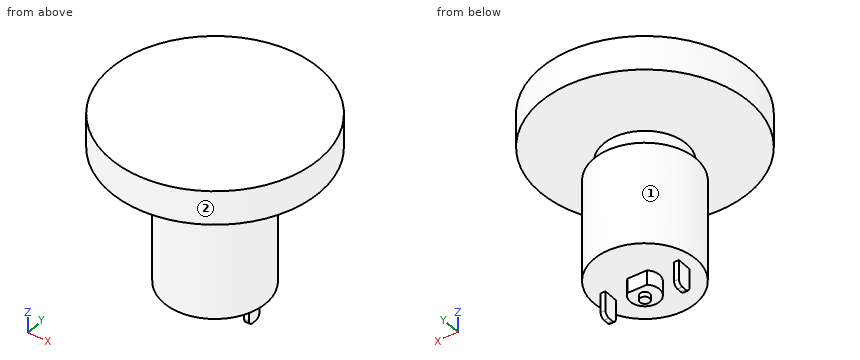
```python
from build123d import *

# Parameters (mm, degrees)
ESQUISSE1_R        = 10.5
BOSS_EXTRU_1_DEPTH = 21
ESQUISSE2_R        = 8.5
BOSS_EXTRU_2_DEPTH = 4
ESQUISSE3_R        = 3
BOSS_EXTRU_3_DEPTH = 2
ESQUISSE4_R        = 1
BOSS_EXTRU_4_DEPTH = 8
ESQUISSE5_W        = 1
ESQUISSE5_H        = 3
BOSS_EXTRU_5_DEPTH = 5
CONG_1_R           = 1
BOSS_EXTRU_6_START = 3
BOSS_EXTRU_6_DEPTH = 3
BOSS_EXTRU_7_START = 1
ESQUISSE7_R        = 1
BOSS_EXTRU_7_DEPTH = 1
ESQUISSE8_R        = 21.5
BOSS_EXTRU_8_DEPTH = 7


with BuildPart() as part:
    # Esquisse1 → Boss.-Extru.1 (new body)
    with BuildSketch(Plane.XY):
        with Locations(Location((-10.784512349, 4.354613187, 0), (0, 0, 180))):
            Circle(ESQUISSE1_R)
    extrude(amount=BOSS_EXTRU_1_DEPTH)

    # Esquisse2 → Boss.-Extru.2 (add)
    with BuildSketch(Plane.XY.offset(21)):
        with Locations((-10.784512349, 4.354613187)):
            Circle(ESQUISSE2_R)
    extrude(amount=BOSS_EXTRU_2_DEPTH)

    # Esquisse3 → Boss.-Extru.3 (add)
    with BuildSketch(Plane.XY.offset(25)):
        with Locations((-10.784512349, 4.354613187)):
            Circle(ESQUISSE3_R)
    extrude(amount=BOSS_EXTRU_3_DEPTH)

    # Esquisse4 → Boss.-Extru.4 (add)
    with BuildSketch(Plane.XY.offset(27)):
        with Locations((-10.784512349, 4.354613187)):
            Circle(ESQUISSE4_R)
    extrude(amount=BOSS_EXTRU_4_DEPTH)

    # Esquisse5 → Boss.-Extru.5 (add)
    with BuildSketch(Plane(origin=(0, 0, 0), x_dir=(-1, 0, 0), z_dir=(0, 0, -1))):
        with Locations((18.284512349, 4.354613187)):
            Rectangle(ESQUISSE5_W, ESQUISSE5_H)
        with Locations((3.284512349, 4.354613187)):
            Rectangle(ESQUISSE5_W, ESQUISSE5_H)
    extrude(amount=BOSS_EXTRU_5_DEPTH)

    # Cong_1
    cong_1_edges = [part.edges().sort_by_distance(p)[0] for p in [
        (-18.284512349, 2.854613187, -5),
        (-18.284512349, 5.854613187, -5),
        (-3.284512349, 5.854613187, -5),
        (-3.284512349, 2.854613187, -5),
    ]]
    fillet(cong_1_edges, radius=CONG_1_R)

    # Esquisse6 → Boss.-Extru.6 (add)
    with BuildSketch(Plane(origin=(0, 0, 0), x_dir=(-1, 0, 0), z_dir=(0, 0, -1)).offset(BOSS_EXTRU_6_START)):
        with BuildLine():
            Line((8.784512349, 6.590681164), (12.784512349, 6.590681164))
            ThreePointArc((12.784512349, 6.590681164), (10.784512349, 1.354613187), (8.784512349, 6.590681164))
        make_face()
    extrude(amount=-BOSS_EXTRU_6_DEPTH)

    # Esquisse7 → Boss.-Extru.7 (add)
    with BuildSketch(Plane(origin=(0, 0, -3), x_dir=(-1, 0, 0), z_dir=(0, 0, -1)).offset(BOSS_EXTRU_7_START)):
        with Locations(Location((10.784512349, 4.354613187, 0), (0, 0, 180))):
            Circle(ESQUISSE7_R)
    extrude(amount=-BOSS_EXTRU_7_DEPTH)

    # Esquisse8 → Boss.-Extru.8 (add)
    with BuildSketch(Plane.XY.offset(35)):
        with Locations((-10.784512349, 4.354613187)):
            Circle(ESQUISSE8_R)
    extrude(amount=-BOSS_EXTRU_8_DEPTH)


solid = part.part
```
The model under review builds one solid part; all positions refer to its coordinate system, in mm. Face numbers are marked on the shaded views. A direction names the side the tool comes from. Round coordinates to 2 decimals unless told otherwise and drop trailing zeros. Order: outer loops, then holes, each group sorted by start corner. A loop starts at its lowest first (then second) coordinate and runs counter-clockwise, first axis right, second up.
Item 1: Add section B-B, the plane x = -1. State the section outline as (y, z) points, and give its area (3 significant figures).
Working result:
outline: (-14.79, 28) - (23.5, 28) - (23.5, 35) - (-14.79, 35) - close; (0.54, 0) - (8.16, 0) - (8.16, 21) - (0.54, 21) - close
area: 428 mm2
Item 2: To check wall thickness, follow probe 1 along Z at (x, y) = (-5.5, -4); probe 2 along Z at (x, y) = (-14, 0); probe 3 along Z at (x, y) = (-26.5, -4.5). State the ranges of each line that lie inside material, in increasing order.
Working result:
probe 1: z = 0 to 21, 28 to 35
probe 2: z = 0 to 25, 28 to 35
probe 3: z = 28 to 35
Item 3: Add section D-D, the plane y = -2. State the section outline as (x, z) points, and give its area (3 significant figures).
Working result:
outline: (-31.32, 28) - (9.75, 28) - (9.75, 35) - (-31.32, 35) - close; (-19.14, 0) - (-2.43, 0) - (-2.43, 21) - (-5.14, 21) - (-5.14, 25) - (-16.43, 25) - (-16.43, 21) - (-19.14, 21) - close
area: 684 mm2
Item 4: Add section C-C, the plane x = -11. State the section outline as (y, z) points.
Working result:
outline: (-17.14, 28) - (3.38, 28) - (3.38, 27) - (1.36, 27) - (1.36, 25) - (-4.14, 25) - (-4.14, 21) - (-6.14, 21) - (-6.14, 0) - (1.36, 0) - (1.36, -3) - (3.38, -3) - (3.38, -4) - (5.33, -4) - (5.33, -3) - (6.59, -3) - (6.59, 0) - (14.85, 0) - (14.85, 21) - (12.85, 21) - (12.85, 25) - (7.35, 25) - (7.35, 27) - (5.33, 27) - (5.33, 28) - (25.85, 28) - (25.85, 35) - (-17.14, 35) - close
Item 5: Machinability: for the marked faces 1 and 2, which of the approach directions +Z, -Z, +X, -X, +Y, -Y give a long, thin tool a straight path to every point of the face, cutting with its end or side? Answer none if there is none.
Working result:
face 1: -Z
face 2: +Z, -Z
Item 6: Add section A-A, the plane y = 10.5. State the section outline as (x, z) points.
Working result:
outline: (-31.39, 28) - (9.82, 28) - (9.82, 35) - (-31.39, 35) - close; (-19.3, 0) - (-2.27, 0) - (-2.27, 21) - (-4.91, 21) - (-4.91, 25) - (-16.66, 25) - (-16.66, 21) - (-19.3, 21) - close
Item 7: For pin 1 (2.5 mm diameter, centred on y = 4, z = -2.5, fed in from -X); pin 2 (3.5 mm diameter, centred on x = -11.5, z = -2, fed in from +Y); pin 3 (0.8 mm diameter, centred on x = -3, z = -2, fed in from +Y), all flat-tipped, find the tip position at first contact; note any pin that passes through.
Working result:
pin 1: stops at x = -18.78
pin 2: stops at y = 6.59
pin 3: stops at y = 5.85
